Input: part model. Units: mm. Frame: model coordinates. A direction names the side the tool comes from. Coordinates: 2 decimals unless noted, no trailing zeros. Order: outer loops, then holes, each group sorted by start corner. A loop starts at its lowest first (then second) coordinate and runs counter-clockwise, first axis right, second up. Notation, with made-up numbers: (26.5, 27.25) -> (55.5, 27.25) arc R26 cw to (55.5, 62.25) -> close; hole circle Ø9 at (76.25, 74.5). An arc over 180 degrees is marked (long way). Answer as CSV lines item,"result".
from build123d import *

# Parameters (mm, degrees)
BASES_R              = 1.95
BASE_DEPTH           = 5.3
SCREWSLOTS_W         = 0.8
SCREWSLOTS_H         = 3.9
SCREWSLOT_DEPTH      = 0.6
MAINSLOT_DEPTH       = 6.97452927
MAINSLOT_DEPTH_BACK  = 6.97452927
MAINSLOTS_W          = 1.95
MAINSLOTS_H          = 2.5
SMALLSLOT_DEPTH      = 6.97452927
SMALLSLOT_DEPTH_BACK = 6.97452927
SMALLSLOTS_W         = 1.95
SMALLSLOTS_H         = 0.9


with BuildPart() as part:
    # BaseS → Base (new body)
    with BuildSketch(Plane(origin=(0, 0, 0), x_dir=(1, 0, 0), z_dir=(0, 1, 0))):
        with Locations(Location((0, 0, 0), (0, 0, 270))):
            Circle(BASES_R)
    extrude(amount=BASE_DEPTH)

    # ScrewSlotS → ScrewSlot (cut)
    with BuildSketch(Plane(origin=(0, 5.3, 0), x_dir=(1, 0, 0), z_dir=(0, 1, 0))):
        Rectangle(SCREWSLOTS_W, SCREWSLOTS_H)
    extrude(amount=-SCREWSLOT_DEPTH, mode=Mode.SUBTRACT)

    # MainSlotS → MainSlot (cut, two sides: drawn at the far end of the back side and taken through both)
    with BuildSketch(Plane.XY.offset(-MAINSLOT_DEPTH_BACK)):
        with Locations((-0.975, 1.85)):
            Rectangle(MAINSLOTS_W, MAINSLOTS_H)
    extrude(amount=MAINSLOT_DEPTH + MAINSLOT_DEPTH_BACK, mode=Mode.SUBTRACT)

    # SmallSlotS → SmallSlot (cut, two sides: drawn at the far end of the back side and taken through both)
    with BuildSketch(Plane(origin=(0, 0, 0), x_dir=(0, 0, -1), z_dir=(1, 0, 0)).offset(-SMALLSLOT_DEPTH_BACK)):
        with Locations((-0.975, 2.65)):
            Rectangle(SMALLSLOTS_W, SMALLSLOTS_H)
    extrude(amount=SMALLSLOT_DEPTH + SMALLSLOT_DEPTH_BACK, mode=Mode.SUBTRACT)

    # O-RingBodyS → O-RingBody (revolve)
    with BuildSketch(Plane.XY):
        Polygon((-1.25, 0), (0, 0), (0, -7.3), (-0.5, -7.3), (-1.5, -6.1), (-1.5, -1.8), (-1.95, -1.8), (-1.95, -1.4), (-1.25, -1.4), align=None)
    revolve(axis=Axis((0, 0, 0), (0, -1, 0)))


solid = part.part
1. Contact query for flat-ended pins moving along their axis: pin 1 (1.5 mm diameter, centred on y = -3, z = 0.5, fed in from -X); pin 2 (1 mm diameter, centred on x = 1, y = 2.5, fed in from +Z); pin 3 (0.7 mm diameter, centred on y = 5, z = 0.5, fed in from -X). Output: stop coordinate, or through.
Findings:
pin 1,"stops at x = -1.5"
pin 2,"stops at z = 1.86"
pin 3,"stops at x = -1.94"
2. Cut plane A-A (y = -1.25). Return the cut outline in (x, z), plus the area to 3 significant figures.
Findings:
outline,"circle Ø2.5 at (0, 0)"
area,"4.91 mm2"
3. Cut plane B-B (y = 3.75). Return the cut outline in (x, z), plus the area to 3 significant figures.
Findings:
outline,"circle Ø3.9 at (0, 0)"
area,"11.9 mm2"
4. Ray query, line 1 along Y through (x, z) = (-1.55, 0.05); line 2 along Y through (x, z) = (1.2, 0.6); line 3 along Y through (x, z) = (1.45, -0.5). Return the intervals inside material, ascending.
Findings:
line 1,"y = -1.8 to -1.4, 0 to 0.6, 3.1 to 5.3"
line 2,"y = -6.29 to -1.4, 0 to 2.2, 3.1 to 5.3"
line 3,"y = -1.8 to -1.4, 0 to 5.3"
5. Mould query, pull axis X, two halves, no side actions, for faces 5 (the face through (1, -1.4, -1)), 6 (the face through (1.933, 2.613, -0.254)), 7 (the face through (0, 4.7, 0)). Classes: released by +X, released by -X, zero draft, split by the parting line, or undercut.
Findings:
face 5,"zero draft"
face 6,"split by the parting line"
face 7,"undercut"
6. Reachability of faces 1 (the face through (1, 2.2, 1)), 2 (the face through (1.5, -3.92, -0.07)), 3 (the face through (-0.5, 3.1, 0.4)), 4 (the face through (0, 2, 0)) from +Z, -Z, +X, -X, +Y, -Y: full face, straight path, thin tool, end or side. Return the list, or none.
Findings:
face 1,"+Z, +X, -X"
face 2,"-Y"
face 3,"+Z, -X"
face 4,"+Z, -Z, -X"
7. Cut plane C-C (y = 0.75). Return the cut outline in (x, z).
Findings:
outline,"(0, -1.95) arc R1.95 ccw to (0, 1.95) -> close"
